The model under review builds one solid part; all positions refer to its coordinate system, in mm. A direction names the side the tool comes from. Give positions to 0.01 mm unless a question says otherwise; leave off trailing zeros. Loops run counter-clockwise (first coordinate to the right, second up) from the corner with the lowest first, then second, coordinate; pieces in that order, holes last. Notation, with made-up numbers: M 26,-12.5 L 31,-12.5 A30 ccw 31,17.5 Z; hole C 82.25,27.5 d7. An arc over 180 degrees is marked long. Return JSON: item names as keys, results as strings. Group by question number.
```python
from build123d import *

# Parameters (mm, degrees)
F0_W      = 190
F0_H      = 5
F1_DEPTH  = 20
F2_W      = 190
F2_H      = 10
F3_DEPTH  = 10
F4_W      = 50
F4_H      = 5
F5_DEPTH  = 70
F7_DEPTH  = 5
F8_W      = 50
F8_H      = 2
F9_DEPTH  = 5.5
F10_W     = 50
F10_H     = 3
F11_DEPTH = 4


with BuildPart() as f1:
    # F0 (on Top) → F1 (new body)
    with BuildSketch(Plane.XY):
        Polygon((0, 20), (0, 0), (5, 0), (5, 5), (5, 15), (5, 20), align=None)
        with Locations((100, 2.5)):
            Rectangle(F0_W, F0_H)
        with Locations((100, 17.5)):
            Rectangle(F0_W, F0_H)
    extrude(amount=F1_DEPTH)

    # F2 (on Top) → F3 (join)
    with BuildSketch(Plane.XY):
        with Locations((100, 10)):
            Rectangle(F2_W, F2_H)
    extrude(amount=F3_DEPTH)

    # F4 (on face) → F5 (join)
    with BuildSketch(Plane.XY.offset(20)):
        with Locations((30, 17.5)):
            Rectangle(F4_W, F4_H)
    extrude(amount=F5_DEPTH)

    # F6 (on face) → F7 (join)
    with BuildSketch(Plane(origin=(0, 20, 0), x_dir=(-1, 0, 0), z_dir=(0, 1, 0))):
        Polygon((-5, 20), (0, 20), (-5, 40), align=None)
        Polygon((-195, 20), (-55, 20), (-55, 40), align=None)
    extrude(amount=-F7_DEPTH)

    # F8 (on face) → F9 (join)
    with BuildSketch(Plane.XY.offset(90)):
        with Locations((30, 19)):
            Rectangle(F8_W, F8_H)
    extrude(amount=F9_DEPTH)

    # F10 (on face) → F11 (join)
    with BuildSketch(Plane.XY.offset(95.5)):
        with Locations((30, 18.5)):
            Rectangle(F10_W, F10_H)
    extrude(amount=F11_DEPTH)


solid = f1.part
```
(1) Add section A-A (x = 32.5). Write out the cut boundary in (y, z).
(2) Add section D-D (x = 98.5). Write out the cut boundary in (y, z), and give its area (3 significant figures).
(3) Mouldability with a two-part tool opening along Y and no side actions: class faces 1 (the flat face through (90, 3, 20)), 2 (the flat face through (30, 17, 97)), 3 (the flat face through (99, 10, 10)), 4 (the flat face through (53, 20, 38)) as released by +Y, released by -Y, zero draft, split by the parting line, or undercut.
(4) Add section B-B (y = 12.75). Write out the cut boundary in (x, z).
(5) Add section C-C (z = 42). Write out the cut boundary in (x, y), and give its area (3 significant figures).
(6) For pin 1 (3 mm diameter, centred on x = 27, z = 97.5, fed in from -Y); pin 2 (4 mm diameter, centred on y = 18.5, z = 75.5, fed in from +X); pin 3 (5 mm diameter, centred on x = 120, y = 10, fed in from +Z), all flat-tipped, find the tip position at first contact; note any pin that passes through.
(7) For faces 5 (the flat face through (99, 5, 15)), 6 (the flat face through (55, 17, 69)), 7 (the flat face through (30, 18, 93)), list the 3-axis set-ups (+Z, -Z, +X, -X, +Y, -Y) from which the entire face can be reached by the end or side of a thin tool; tool diameter is ignored.
(8) For probe 1 along Z at (x, y) = (50, 3); probe 2 along Z at (x, y) = (73.5, 13.75); probe 3 along X at (y, z) = (17.75, 57), list the stretches that pass through material, from the lowest coordinate up.
Verdict:
{
 "1": {"outline": "M 0,0 L 20,0 L 20,99.5 L 17,99.5 L 17,95.5 L 18,95.5 L 18,90 L 15,90 L 15,10 L 5,10 L 5,20 L 0,20 Z"},
 "2": {"outline": "M 0,0 L 20,0 L 20,33.79 L 15,33.79 L 15,10 L 5,10 L 5,20 L 0,20 Z", "area": "369 mm²"},
 "3": {"face 1": "zero draft", "face 2": "released by -Y", "face 3": "undercut", "face 4": "released by +Y"},
 "4": {"outline": "M 0,0 L 195,0 L 195,10 L 5,10 L 5,20 L 0,20 Z"},
 "5": {"outline": "M 5,15 L 55,15 L 55,20 L 5,20 Z", "area": "250 mm²"},
 "6": {"pin 1": "stops at y = 17", "pin 2": "stops at x = 55", "pin 3": "stops at z = 10"},
 "7": {"face 5": "+Z, +X", "face 6": "+Z, +X, +Y, -Y", "face 7": "+X, -X, -Y"},
 "8": {"probe 1": "z = 0 to 20", "probe 2": "z = 0 to 10", "probe 3": "x = 5 to 55"}
}
